Build history of the part. All positions in model axes, mm. Round coordinates to 2 decimals unless told otherwise and drop trailing zeros.
1) Pull direction X, two halves, no side cores. Call faces 1 (the cylindrical face through (41.37, 1.48, 96.66)), 2 (the flat face through (1, 0, 1)): +X half, -X half, draft (parallel to the pull), parting line (faces both ways), or undercut.
2) Flat gauge pin, fed straight in: pin 1 (1.9 mm diameter, centred on x = 1.89, z = 7.23, fed in from -Y). Where does the tip first touch, or does it go through?
3) Wall check: probe 1 along Z at (x, y) = (-41, 2.4); probe 2 along X at (y, z) = (2.4, 15); probe 3 along Z at (x, y) = (1, 0.45). Give the ranges that are in metal, low to high.
Autodesk Inventor part; units mm, degrees
ref_plane "YZ Plane" through (0, 0, 0) normal (1, 0, 0) x (0, 1, 0)
ref_plane "XZ Plane" through (0, 0, 0) normal (0, 1, 0) x (-1, 0, 0)
ref_plane "XY Plane" through (0, 0, 0) normal (0, 0, 1) x (1, 0, 0)
sketch "Skizze1" plane through (0, 0, 0) normal (0, 1, 0) x (-1, 0, 0)
  line L0 (45, 100) -> (45, -100)
  line L1 (45, -100) -> (-45, -100)
  line L2 (-45, -100) -> (-45, 100)
  line L3 (-45, 100) -> (45, 100)
  line L4 (0, 61.8387) -> (0, -129.7607) construction
  line L5 (83.0665, 0) -> (-88.5254, 0) construction
  circle A0 centre (41, 95) radius 1.7
  circle A1 centre (-41, 95) radius 1.7
  circle A2 centre (-41, -95) radius 1.7
  circle A3 centre (41, -95) radius 1.7
  circle A4 centre (3.1127, 7.2251) radius 1.5558
  circle A5 centre (3.1127, -8.3324) radius 1.5558
  circle A6 centre (-41, 15) radius 1.7
  circle A7 centre (41, 15) radius 1.7
  circle A8 centre (-41, -65) radius 1.7
  circle A9 centre (41, -65) radius 1.7
  circle A10 centre (-41, -145) radius 1.7
  circle A11 centre (41, -145) radius 1.7
  circle A12 centre (-41, -225) radius 1.7
  circle A13 centre (41, -225) radius 1.7
  circle A14 centre (-41, -305) radius 1.7
  circle A15 centre (41, -305) radius 1.7
  circle A16 centre (-41, -385) radius 1.7
  circle A17 centre (41, -385) radius 1.7
  circle A18 centre (-41, -465) radius 1.7
  circle A19 centre (41, -465) radius 1.7
  circle A20 centre (-41, -545) radius 1.7
  circle A21 centre (41, -545) radius 1.7
  circle A22 centre (-41, -625) radius 1.7
  circle A23 centre (41, -625) radius 1.7
  circle A24 centre (-41, -705) radius 1.7
  circle A25 centre (41, -705) radius 1.7
  circle A26 centre (-41, -785) radius 1.7
  circle A27 centre (41, -785) radius 1.7
  circle A28 centre (-41, -865) radius 1.7
  circle A29 centre (41, -865) radius 1.7
  circle A30 centre (-41, -945) radius 1.7
  circle A31 centre (41, -945) radius 1.7
  circle A32 centre (-41, -1025) radius 1.7
  circle A33 centre (41, -1025) radius 1.7
  circle A34 centre (-41, -1105) radius 1.7
  circle A35 centre (41, -1105) radius 1.7
  circle A36 centre (-41, -1185) radius 1.7
  circle A37 centre (41, -1185) radius 1.7
  circle A38 centre (-41, -1265) radius 1.7
  circle A39 centre (41, -1265) radius 1.7
  circle A40 centre (-41, -1345) radius 1.7
  circle A41 centre (41, -1345) radius 1.7
  circle A42 centre (-41, -1425) radius 1.7
  circle A43 centre (41, -1425) radius 1.7
  circle A44 centre (-41, -1505) radius 1.7
  circle A45 centre (41, -1505) radius 1.7
  circle A46 centre (-41, -1585) radius 1.7
  circle A47 centre (41, -1585) radius 1.7
  circle A48 centre (-41, -1665) radius 1.7
  circle A49 centre (41, -1665) radius 1.7
  circle A50 centre (-41, -1745) radius 1.7
  circle A51 centre (41, -1745) radius 1.7
  circle A52 centre (-41, -1825) radius 1.7
  circle A53 centre (41, -1825) radius 1.7
  circle A54 centre (-41, -1905) radius 1.7
  circle A55 centre (41, -1905) radius 1.7
  circle A56 centre (-41, -1985) radius 1.7
  circle A57 centre (41, -1985) radius 1.7
  circle A58 centre (-41, -2065) radius 1.7
  circle A59 centre (41, -2065) radius 1.7
  circle A60 centre (-41, -2145) radius 1.7
  circle A61 centre (41, -2145) radius 1.7
  circle A62 centre (-41, -2225) radius 1.7
  circle A63 centre (41, -2225) radius 1.7
  circle A64 centre (-41, -2305) radius 1.7
  circle A65 centre (41, -2305) radius 1.7
  circle A66 centre (-41, -2385) radius 1.7
  circle A67 centre (41, -2385) radius 1.7
  circle A68 centre (-41, -2465) radius 1.7
  circle A69 centre (41, -2465) radius 1.7
  circle A70 centre (-41, -2545) radius 1.7
  circle A71 centre (41, -2545) radius 1.7
  circle A72 centre (-41, -2625) radius 1.7
  circle A73 centre (41, -2625) radius 1.7
  circle A74 centre (-41, -2705) radius 1.7
  circle A75 centre (41, -2705) radius 1.7
  circle A76 centre (-41, -2785) radius 1.7
  circle A77 centre (41, -2785) radius 1.7
  circle A78 centre (-41, -2865) radius 1.7
  circle A79 centre (41, -2865) radius 1.7
  circle A80 centre (-41, -2945) radius 1.7
  circle A81 centre (41, -2945) radius 1.7
  circle A82 centre (-41, -3025) radius 1.7
  circle A83 centre (41, -3025) radius 1.7
  circle A84 centre (-41, -3105) radius 1.7
  circle A85 centre (41, -3105) radius 1.7
  circle A86 centre (-41, -3185) radius 1.7
  circle A87 centre (41, -3185) radius 1.7
  circle A88 centre (-41, -3265) radius 1.7
  circle A89 centre (41, -3265) radius 1.7
  circle A90 centre (-41, -3345) radius 1.7
  circle A91 centre (41, -3345) radius 1.7
  circle A92 centre (-41, -3425) radius 1.7
  circle A93 centre (41, -3425) radius 1.7
  circle A94 centre (-41, -3505) radius 1.7
  circle A95 centre (41, -3505) radius 1.7
  circle A96 centre (-41, -3585) radius 1.7
  circle A97 centre (41, -3585) radius 1.7
  circle A98 centre (-41, -3665) radius 1.7
  circle A99 centre (41, -3665) radius 1.7
  circle A100 centre (-41, -3745) radius 1.7
  circle A101 centre (41, -3745) radius 1.7
  circle A102 centre (-41, -3825) radius 1.7
  circle A103 centre (41, -3825) radius 1.7
  circle A104 centre (-41, -3905) radius 1.7
  circle A105 centre (41, -3905) radius 1.7
  circle A106 centre (-41, -3985) radius 1.7
  circle A107 centre (41, -3985) radius 1.7
  circle A108 centre (-41, -4065) radius 1.7
  circle A109 centre (41, -4065) radius 1.7
  circle A110 centre (-41, -4145) radius 1.7
  circle A111 centre (41, -4145) radius 1.7
  circle A112 centre (-41, -4225) radius 1.7
  circle A113 centre (41, -4225) radius 1.7
  circle A114 centre (-41, -4305) radius 1.7
  circle A115 centre (41, -4305) radius 1.7
  circle A116 centre (-41, -4385) radius 1.7
  circle A117 centre (41, -4385) radius 1.7
  circle A118 centre (-41, -4465) radius 1.7
  circle A119 centre (41, -4465) radius 1.7
  circle A120 centre (-41, -4545) radius 1.7
  circle A121 centre (41, -4545) radius 1.7
  circle A122 centre (-41, -4625) radius 1.7
  circle A123 centre (41, -4625) radius 1.7
  circle A124 centre (-41, -4705) radius 1.7
  circle A125 centre (41, -4705) radius 1.7
  circle A126 centre (-41, -4785) radius 1.7
  circle A127 centre (41, -4785) radius 1.7
  circle A128 centre (-41, -4865) radius 1.7
  circle A129 centre (41, -4865) radius 1.7
  circle A130 centre (-41, -4945) radius 1.7
  circle A131 centre (41, -4945) radius 1.7
  circle A132 centre (-41, -5025) radius 1.7
  circle A133 centre (41, -5025) radius 1.7
  circle A134 centre (-41, -5105) radius 1.7
  circle A135 centre (41, -5105) radius 1.7
  circle A136 centre (-41, -5185) radius 1.7
  circle A137 centre (41, -5185) radius 1.7
  circle A138 centre (-41, -5265) radius 1.7
  circle A139 centre (41, -5265) radius 1.7
  circle A140 centre (-41, -5345) radius 1.7
  circle A141 centre (41, -5345) radius 1.7
  circle A142 centre (-41, -5425) radius 1.7
  circle A143 centre (41, -5425) radius 1.7
  circle A144 centre (-41, -5505) radius 1.7
  circle A145 centre (41, -5505) radius 1.7
  circle A146 centre (-41, -5585) radius 1.7
  circle A147 centre (41, -5585) radius 1.7
  circle A148 centre (-41, -5665) radius 1.7
  circle A149 centre (41, -5665) radius 1.7
  circle A150 centre (-41, -5745) radius 1.7
  circle A151 centre (41, -5745) radius 1.7
  circle A152 centre (-41, -5825) radius 1.7
  circle A153 centre (41, -5825) radius 1.7
  circle A154 centre (-41, -5905) radius 1.7
  circle A155 centre (41, -5905) radius 1.7
  circle A156 centre (-41, -5985) radius 1.7
  circle A157 centre (41, -5985) radius 1.7
  circle A158 centre (-41, -6065) radius 1.7
  circle A159 centre (41, -6065) radius 1.7
  circle A160 centre (-41, -6145) radius 1.7
  circle A161 centre (41, -6145) radius 1.7
  circle A162 centre (-41, -6225) radius 1.7
  circle A163 centre (41, -6225) radius 1.7
  circle A164 centre (-41, -35) radius 1.7
  circle A165 centre (41, -35) radius 1.7
  point P0 (0, 0)
  dimension "d1" = 45
  dimension "d2" = 45
  dimension "d3" = 100
  dimension "d4" = 100
  dimension "d7" = 3.4
  dimension "d8" = 4
  dimension "d9" = 5
  dimension "d10" = 3.4
  dimension "d11" = 4
  dimension "d12" = 5
  dimension "d13" = 3.4
  dimension "d14" = 4
  dimension "d15" = 5
  dimension "d16" = 3.4
  dimension "d17" = 5
  dimension "d18" = 4
  dimension "d25" = 80
  dimension "d32" = 50
extrude "Extrusion1" add sketch "Skizze1" along normal blind 3 contours L0 L1 L2 L3 | A0 | A1 | A2 | A3 | A4 | A5 | A6 | A7 | A8 | A9 | A164 | A165
extrude "Extrusion2" cut sketch "Skizze1" along normal blind 10 contours A0 | A1 | A2 | A3 | A6 | A7 | A164 | A165
sketch "Skizze2" plane through (0, 0, 0) normal (0, -1, 0) x (1, 0, 0)
  circle A0 centre (1.8873, 7.2251) radius 1.5557
  circle A1 centre (1.8873, -8.3324) radius 1.5557
  point P0 (0, 0)
extrude "Extrusion3" cut sketch "Skizze2" against normal blind 10
properties part number "Chassis-2" material "CFK"
Evaluation:
1. face 1: undercut
1. face 2: draft
2. pin 1: passes through
3. probe 1: z = -100 to -96.7, -93.3 to -36.7, -33.3 to 13.3, 16.7 to 93.3, 96.7 to 100
3. probe 2: x = -45 to -42.7, -39.3 to 39.3, 42.7 to 45
3. probe 3: z = -100 to -9.61, -7.05 to 5.95, 8.5 to 100
